Could you check a few things on this drawing? It's one solid part, dimensions in mm from its lowest x, y, z. Coordinates: 2 decimals unless noted, no trailing zeros. Write each loop counter-clockwise with the first axis right and the second up, starting at its lowest first coordinate (ties: lowest second). Pieces come first, ordered by that corner, then holes. Notation, with made-up numbers: (62.5, 38.5) - (106.5, 38.5) arc R9 ccw to (106.5, 52.5) - close; hole circle Ø10 at (24, -16). An arc over 180 degrees is marked (long way). Use one line per item in the form item = value. Start each with the question number.
(1) For pin 1 Ø2 at (x, z) = (16.5, 2) entering from +Y; pin 2 Ø6 at (x, y) = (8, 14) entering from +Z; pin 3 Ø0.5 at (x, z) = (13.5, 1) entering from -Y, each with a flat end and sliding along its axis, tell me the tip position at first contact or that it passes through.
(2) If we section it at B-B on z = 0.5: Please give me the cut outline in (x, y), then the cut area to 3 significant figures.
(3) Thinking about a two-plate mould opening in Y: for the marked faces 1 and 2, which applies, pulls with the +Y half, pulls with the -Y half, needs draft (parallel to the pull), parting line crosses it, or undercut?
(4) If we section it at C-C on x = 4: Please give me the cut outline in (y, z), then the cut area to 3 significant figures.
(5) If we section it at D-D on y = 8.1: Please give me the cut outline in (x, z).
(6) If I drill on probe 1 along Y at (x, z) = (1.8, 1.05); probe 2 along Z at (x, y) = (16.25, 22.5); probe 3 along Y at (x, z) = (6, 4.75), over which ranges is the centre line in solid material (lowest first)? Write a range as from..to.
(7) If we section it at A-A on x = 20: Please give me the cut outline in (y, z).
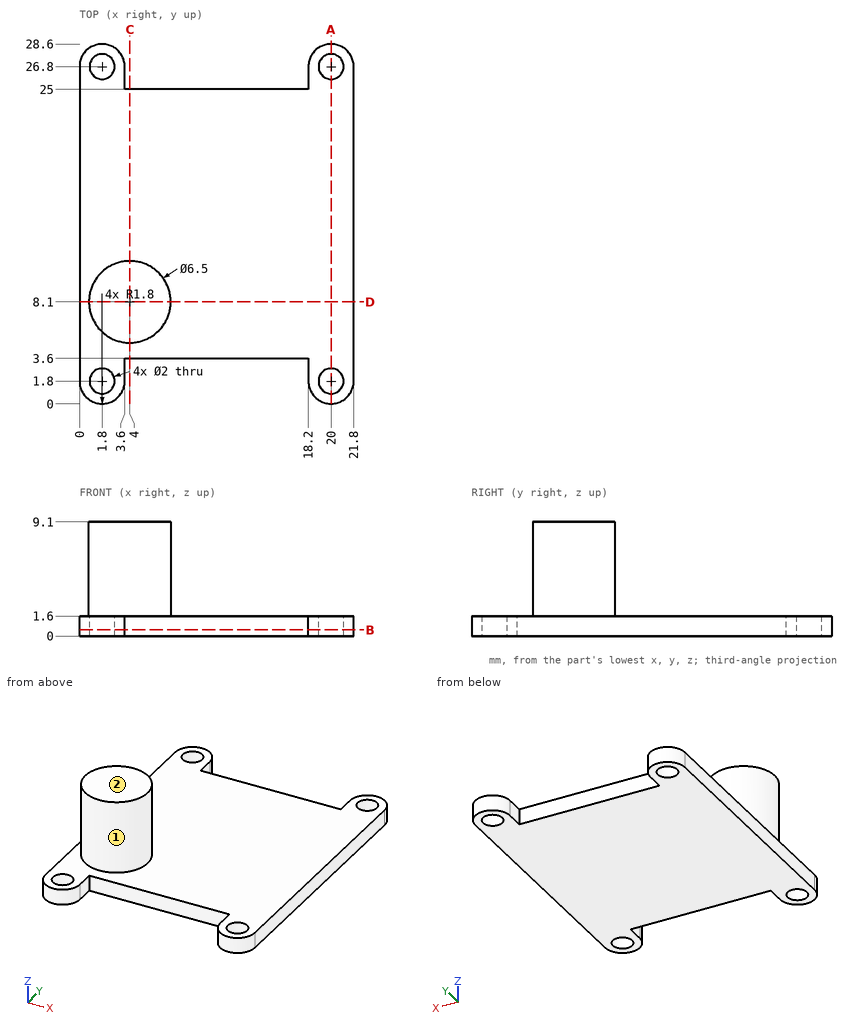
Reported:
q1.pin_1 = 25
q1.pin_2 = 1.6
q1.pin_3 = 3.6
q2.outline = (0, 1.8) arc R1.8 ccw to (3.6, 1.8) - (3.6, 3.6) - (18.2, 3.6) - (18.2, 1.8) arc R1.8 ccw to (21.8, 1.8) - (21.8, 26.8) arc R1.8 ccw to (18.2, 26.8) - (18.2, 25) - (3.6, 25) - (3.6, 26.8) arc R1.8 ccw to (0, 26.8) - close; hole circle Ø2 at (1.8, 1.8); hole circle Ø2 at (1.8, 26.8); hole circle Ø2 at (20, 1.8); hole circle Ø2 at (20, 26.8)
q2.area = 500 mm2
q3.face_1 = parting line crosses it
q3.face_2 = needs draft
q4.outline = (3.6, 0) - (25, 0) - (25, 1.6) - (11.35, 1.6) - (11.35, 9.1) - (4.85, 9.1) - (4.85, 1.6) - (3.6, 1.6) - close
q4.area = 83.0 mm2
q5.outline = (0, 0) - (21.8, 0) - (21.8, 1.6) - (7.25, 1.6) - (7.25, 9.1) - (0.75, 9.1) - (0.75, 1.6) - (0, 1.6) - close
q6.probe_1 = 0..0.8, 2.8..25.8, 27.8..28.6
q6.probe_2 = 0..1.6
q6.probe_3 = 5.54..10.66
q7.outline = (0, 0) - (0.8, 0) - (0.8, 1.6) - (0, 1.6) - close; (2.8, 0) - (25.8, 0) - (25.8, 1.6) - (2.8, 1.6) - close; (27.8, 0) - (28.6, 0) - (28.6, 1.6) - (27.8, 1.6) - close
